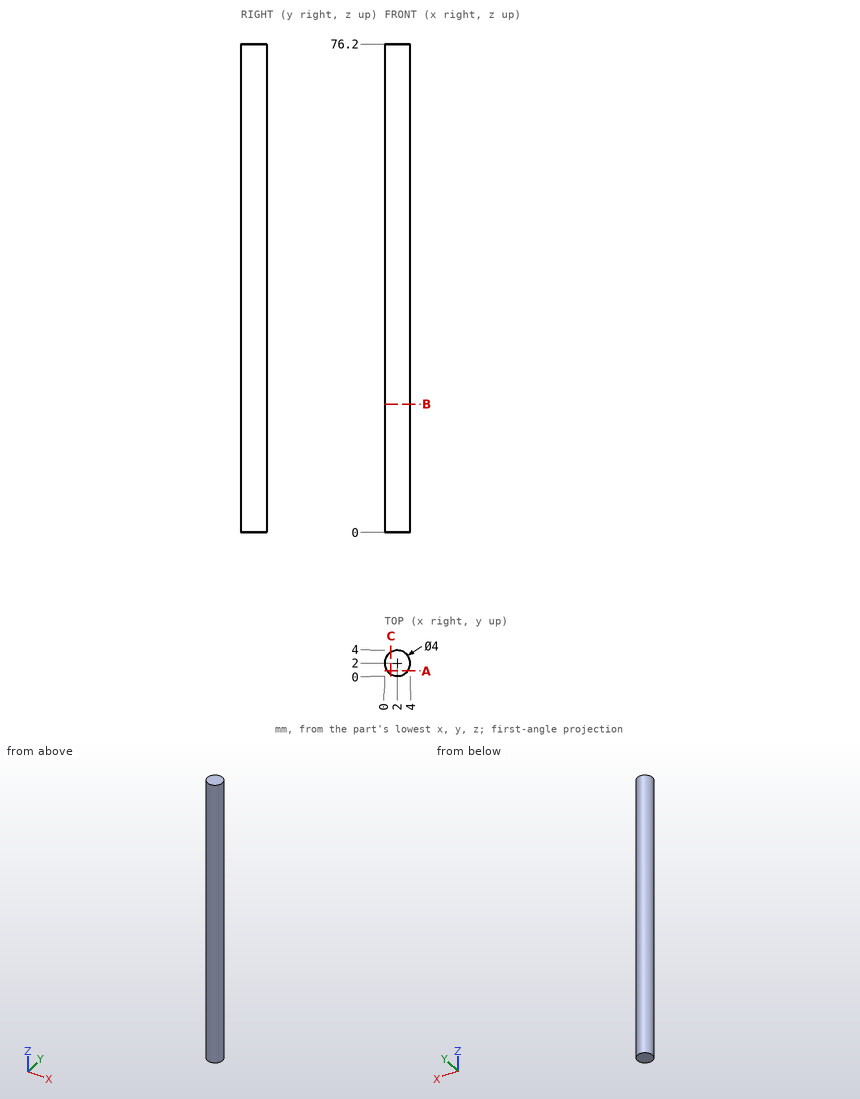
Print and shaded views of the part. All mm, measured from the part's lowest x, y and z. Round coordinates to 2 decimals unless told otherwise and drop trailing zeros. Write each loop counter-clockwise with the first axis right and the second up, starting at its lowest first coordinate (ties: lowest second). Pieces come first, ordered by that corner, then holes. Notation, with made-up numbers: (-18, -26) -> (16, -26) arc R36 ccw to (16, 8) -> close; hole circle Ø8 at (45.25, 65). An arc over 180 degrees is marked (long way). Write item = value, one per line.
(1) Band-saw the part on C-C (x = 1). Give the cut face in (y, z), then the cut area to 3 significant figures.
Answer:
outline = (0.27, 0) -> (3.73, 0) -> (3.73, 76.2) -> (0.27, 76.2) -> close
area = 264 mm2
(2) Band-saw the part on B-B (z = 20). Give the cut face in (x, y).
Answer:
outline = circle Ø4 at (2, 2)
(3) Probe L1, parallel to Y at x = 1.9, z = 21; L2, parallel to Y at x = 2.5, z = 26. List the from-to ranges inside material, lowest first.
Answer:
L1 = 0 to 4
L2 = 0.06 to 3.94
(4) Band-saw the part on A-A (y = 0.8). Give the cut face in (x, z), then the cut area to 3 significant figures.
Answer:
outline = (0.4, 0) -> (3.6, 0) -> (3.6, 76.2) -> (0.4, 76.2) -> close
area = 244 mm2
